Design review of the part built by this model. Coordinates are the model's own, in mm. A direction names the side the tool comes from. Round coordinates to 2 decimals unless told otherwise and drop trailing zeros. Write each loop counter-clockwise with the first axis right and the second up, starting at its lowest first coordinate (ties: lowest second). Pieces come first, ordered by that corner, then holes.
from build123d import *

# Parameters (mm, degrees)
ESQUISSE1_W              = 30
ESQUISSE1_H              = 50
BOSS_EXTRU_1_DEPTH       = 40
BOSS_EXTRU_3_START       = -40
BOSS_EXTRU_3_OUTLINE_R   = 7.75
BOSS_EXTRU_3_DEPTH       = 40
ESQUISSE138_W            = 14
ESQUISSE138_H            = 8.5
BOSS_EXTRU_4_DEPTH       = 55
ESQUISSE145_W            = 8
ESQUISSE145_H            = 4
BOSS_EXTRU_5_DEPTH       = 10
ESQUISSE146_R            = 2.3
ENL_V_MAT_EXTRU_13_DEPTH = 39
ESQUISSE147_W            = 3
ESQUISSE147_H            = 6.5
ENL_V_MAT_EXTRU_14_DEPTH = 40
ESQUISSE150_W            = 10
ESQUISSE150_H            = 8.2
BOSS_EXTRU_6_DEPTH       = 12
ESQUISSE154_W            = 14
ESQUISSE154_H            = 16
BOSS_EXTRU_7_DEPTH       = 23
ESQUISSE152_R            = 3.5
ENL_V_MAT_EXTRU_16_DEPTH = 40


# Read off the part's stored shape, not the designer's step: Boss.-Extru.3
with BuildPart() as part:
    # Esquisse1 → Boss.-Extru.1 (new body)
    with BuildSketch(Plane.XY):
        with Locations((15, 25)):
            Rectangle(ESQUISSE1_W, ESQUISSE1_H)
    extrude(amount=BOSS_EXTRU_1_DEPTH)

    # Boss.-Extru.3 outline → Boss.-Extru.3 (cut)
    with BuildSketch(Plane.XY.offset(40).offset(BOSS_EXTRU_3_START)):
        with Locations((15, 12.3)):
            Circle(BOSS_EXTRU_3_OUTLINE_R)
        with Locations((15, 37.7)):
            Circle(BOSS_EXTRU_3_OUTLINE_R)
    extrude(amount=BOSS_EXTRU_3_DEPTH, mode=Mode.SUBTRACT)

    # Esquisse138 → Boss.-Extru.4 (add)
    with BuildSketch(Plane(origin=(0, 50, 0), x_dir=(1, 0, 0), z_dir=(0, 1, 0))):
        with Locations((23, -35.75)):
            Rectangle(ESQUISSE138_W, ESQUISSE138_H)
        with Locations((23, -4.25)):
            Rectangle(ESQUISSE138_W, ESQUISSE138_H)
    extrude(amount=BOSS_EXTRU_4_DEPTH)

    # Esquisse145 → Boss.-Extru.5 (add)
    with BuildSketch(Plane(origin=(30, 0, 0), x_dir=(0, 0, -1), z_dir=(1, 0, 0))):
        with Locations((-32, 48)):
            Rectangle(ESQUISSE145_W, ESQUISSE145_H)
        with Locations((-8, 48)):
            Rectangle(ESQUISSE145_W, ESQUISSE145_H)
        with Locations((-32, 28)):
            Rectangle(ESQUISSE145_W, ESQUISSE145_H)
        with Locations((-8, 28)):
            Rectangle(ESQUISSE145_W, ESQUISSE145_H)
    extrude(amount=BOSS_EXTRU_5_DEPTH)

    # Esquisse146 → Enlèv. mat.-Extru.13 (cut)
    with BuildSketch(Plane(origin=(0, 50, 0), x_dir=(1, 0, 0), z_dir=(0, 1, 0))):
        with Locations(Location((36, -32, 0), (0, 0, 270))):
            Circle(ESQUISSE146_R)
        with Locations(Location((36, -8, 0), (0, 0, 270))):
            Circle(ESQUISSE146_R)
    extrude(amount=-ENL_V_MAT_EXTRU_13_DEPTH, mode=Mode.SUBTRACT)

    # Esquisse147 → Enlèv. mat.-Extru.14 (cut)
    with BuildSketch(Plane.XY.offset(40)):
        with Locations((20, 68.25)):
            Rectangle(ESQUISSE147_W, ESQUISSE147_H)
    extrude(amount=-ENL_V_MAT_EXTRU_14_DEPTH, mode=Mode.SUBTRACT)

    # Esquisse150 → Boss.-Extru.6 (add)
    with BuildSketch(Plane(origin=(0, 50, 0), x_dir=(1, 0, 0), z_dir=(0, 1, 0))):
        with Locations((9, -4.1)):
            Rectangle(ESQUISSE150_W, ESQUISSE150_H)
        with Locations((9, -35.9)):
            Rectangle(ESQUISSE150_W, ESQUISSE150_H)
    extrude(amount=BOSS_EXTRU_6_DEPTH)

    # Esquisse154 → Boss.-Extru.7 (add)
    with BuildSketch(Plane.XY.offset(8.5)):
        with Locations((23, 97)):
            Rectangle(ESQUISSE154_W, ESQUISSE154_H)
    extrude(amount=BOSS_EXTRU_7_DEPTH)

    # Esquisse152 → Enlèv. mat.-Extru.16 (cut)
    with BuildSketch(Plane.XY.offset(40)):
        with Locations((23, 95)):
            Circle(ESQUISSE152_R)
    extrude(amount=-ENL_V_MAT_EXTRU_16_DEPTH, mode=Mode.SUBTRACT)


solid = part.part
1) For faces 4 (the face through (15, 50, 20)), 5 (the face through (23, 89, 20)), 6 (the face through (33, 26, 32)), 7 (the face through (33, 30, 32)), 8 (the face through (18.5, 68, 36)), list the 3-axis set-ups (+Z, -Z, +X, -X, +Y, -Y) from which the entire face can be reached by the end or side of a thin tool; tool diameter is ignored.
2) Add section B-B on y = 95. State the section outline as (x, z) points, and give its area (3 significant figures).
3) Add section C-C on x = 17.5. State the section outline as (y, z) points, and give its area (3 significant figures).
4) For P1, Ø4, axis at y = 57.5, z = 34, coming from the +X side; P2, Ø6.5, axis at x = 33.5, z = 33, coming from the +Y side; P3, Ø9, axis at y = 55.5, z = 35.5, coming from the -X side, all flat-tipped, find the tip position at first contact; note any pin that passes through.
5) For line 1 along Y through (x, z) = (23, 24); line 2 along Y through (x, z) = (24, 11.5); line 3 along Z through (x, y) = (16.5, 86.5), list the stretches that pass through material, from the lowest coordinate up.
6) Add section D-D on x = 36. Count the separate pieces of the cut face and the enclosed holes in it, and give its area (3 significant figures).
7) Add section A-A on z = 26.5. State the section outline as (x, y) points, and give its area (3 significant figures).
8) The part is to be moulded in two halves that separate along X. For faces 1 (the face through (22.241, 91.583, 20.28)), 2 (the face through (35, 28, 4)), 3 (the face through (40, 48, 32)), say which applies: pulls with the +X half, pulls with the -X half, needs draft (parallel to the pull), parting line crosses it, or undercut.
Computed:
1. face 4: none
1. face 5: +X, -X
1. face 6: +Z, -Z, +X, -Y
1. face 7: +Z, -Z, +X
1. face 8: +Z, -Z
2. outline: (16, 0) - (19.5, 0) - (19.5, 40) - (16, 40) - close; (26.5, 0) - (30, 0) - (30, 40) - (26.5, 40) - close
2. area: 280 mm2
3. outline: (0, 0) - (4.96, 0) - (4.96, 40) - (0, 40) - close; (19.64, 0) - (30.36, 0) - (30.36, 40) - (19.64, 40) - close; (45.04, 0) - (105, 0) - (105, 40) - (45.04, 40) - close; hole (50, 8.5) - (89, 8.5) - (89, 31.5) - (50, 31.5) - close
3. area: 2,130 mm2
4. P1: stops at x = 30
4. P2: stops at y = 50
4. P3: stops at x = 4
5. line 1: y = 0 to 50, 89 to 91.5, 98.5 to 105
5. line 2: y = 0 to 50, 89 to 91.65, 98.35 to 105
5. line 3: z = 0 to 8.5, 31.5 to 40
6. separate pieces: 8
6. enclosed holes: 0
6. area: 54.4 mm2
7. outline: (0, 0) - (30, 0) - (30, 50) - (0, 50) - close; (16, 89) - (30, 89) - (30, 105) - (16, 105) - close; hole circle Ø15.5 at (15, 12.3); hole circle Ø15.5 at (15, 37.7); hole circle Ø7 at (23, 95)
7. area: 1,310 mm2
8. face 1: undercut
8. face 2: needs draft
8. face 3: pulls with the +X half
